Geometry: final body of the model. Coordinates: model frame, mm. Face numbers are marked on the shaded views. A direction names the side the tool comes from. Round coordinates to 2 decimals unless told otherwise and drop trailing zeros. Order: outer loops, then holes, each group sorted by start corner. A loop starts at its lowest first (then second) coordinate and runs counter-clockwise, first axis right, second up. Notation, with made-up numbers: M 82.5,84.5 L 105.5,84.5 A20 cw 105.5,100.5 Z; hole C 32.5,75.25 d6. An arc over 180 degrees is marked long. Put each result on its own line as item: value. Start each with the question number.
1) Access query for the marked faces 1, 2 and 3. Directions: +Z, -Z, +X, -X, +Y, -Y. A direction counts if a zero-diameter tool reaches every point of the face in a straight line with its end or side. Return the directions, or none.
2) Material intervals for probe 1 along Y at (x, z) = (3.5, 1.2); probe 2 along X at (y, z) = (17.5, 0.6); probe 3 along X at (y, z) = (-14.5, 3.15), sorted ascending. Write a range as [from, to].
3) Draft query along X for the marked faces 4, 5 and 6. Return one class per face: pulls with the +X half, pulls with the -X half, needs draft (parallel to the pull), parting line crosses it, or undercut.
4) Section A-A, the plane x = -6.5. Return loops of the section in (y, z), then the cut area to 3 significant figures.
5) First-contact query: P1, Ø2.5, axis at x = -7.5, z = 3.5, coming from the +Y side; P2, Ø2.5, axis at x = -4.5, z = 1.5, coming from the -Y side; P3, Ø2.5, axis at y = 9.5, z = 2, coming from the -X side. Flat tips, straight axial feed; report the tip coordinate or a pass-through.
6) Section C-C, the plane z = 2.2. Return loops of the section in (x, y).
7) Section B-B, the plane y = 5.5. Return loops of the section in (x, z).
Autodesk Inventor part; units mm, degrees
ref_plane "YZ Plane" through (0, 0, 0) normal (1, 0, 0) x (0, 1, 0)
ref_plane "XZ Plane" through (0, 0, 0) normal (0, 1, 0) x (-1, 0, 0)
ref_plane "XY Plane" through (0, 0, 0) normal (0, 0, 1) x (1, 0, 0)
sketch "Sketch1" plane through (0, 0, 0) normal (0, 0, 1) x (1, 0, 0)
  line L0 (-20, 24) -> (20, 24)
  line L1 (20, 24) -> (20, -24)
  line L2 (20, -24) -> (-20, -24)
  line L3 (-20, -24) -> (-20, 24)
  line L4 (-14.25, 19) -> (14.25, 19)
  line L5 (14.25, 19) -> (14.25, -9.5)
  line L6 (14.25, -9.5) -> (-14.25, -9.5)
  line L7 (-14.25, -9.5) -> (-14.25, 19)
  circle A0 centre (-20, 24) radius 4
  circle A1 centre (20, 24) radius 4
  circle A2 centre (20, -24) radius 4
  circle A3 centre (-20, -24) radius 4
  point P0 (20, 0)
  point P1 (0, 24)
  point P2 (0, 0)
  point P3 (-20, 0)
  point P4 (0, 19)
  dimension "d0" = 40
  dimension "d1" = 48
  dimension "d3" = 5
  dimension "d4" = 28.5
  dimension "d5" = 28.5
  dimension "d8" = 8
  dimension "d9" = 8
  dimension "d10" = 8
  dimension "d11" = 8
extrude "Extrusion1" add sketch "Sketch1" along normal blind 5
properties part number "cubierta OLED"
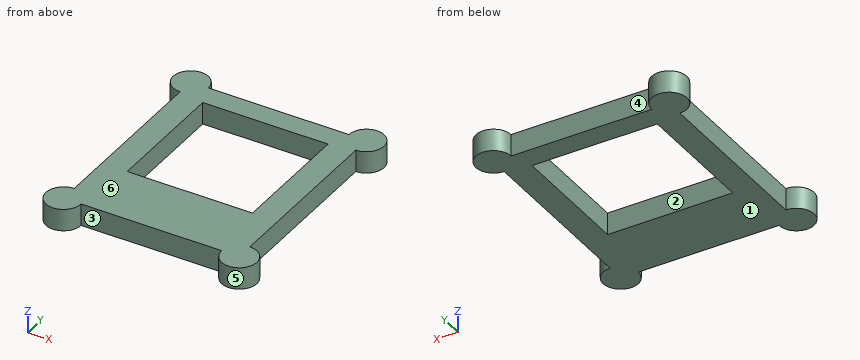
Result sheet:
1. face 1: -Z, +X, -X, +Y, -Y
1. face 2: +Z, -Z
1. face 3: +Z, -Z, -Y
2. probe 1: y = [-24, -9.5], [19, 24]
2. probe 2: x = [-20, -14.25], [14.25, 20]
2. probe 3: x = [-20, 20]
3. face 4: undercut
3. face 5: undercut
3. face 6: needs draft
4. outline: M -24,0 L -9.5,0 L -9.5,5 L -24,5 Z; M 19,0 L 24,0 L 24,5 L 19,5 Z
4. area: 97.5 mm2
5. P1: stops at y = 24
5. P2: stops at y = -24
5. P3: stops at x = -20
6. outline: M -20,-20 A4 ccw long -16,-24 L 16,-24 A4 ccw long 20,-20 L 20,20 A4 ccw long 16,24 L -16,24 A4 ccw long -20,20 Z; hole M -14.25,-9.5 L 14.25,-9.5 L 14.25,19 L -14.25,19 Z
7. outline: M -20,0 L -14.25,0 L -14.25,5 L -20,5 Z; M 14.25,0 L 20,0 L 20,5 L 14.25,5 Z
